Autodesk Inventor part; units mm, degrees
ref_plane "YZ Plane" through (0, 0, 0) normal (1, 0, 0) x (0, 1, 0)
ref_plane "XZ Plane" through (0, 0, 0) normal (0, 1, 0) x (-1, 0, 0)
ref_plane "XY Plane" through (0, 0, 0) normal (0, 0, 1) x (1, 0, 0)
sketch "Skizze1" plane through (0, 0, 0) normal (0, 0, 1) x (1, 0, 0)
  line L0 (0, 0) -> (15, 0)
  line L1 (15, 0) -> (15, -25)
  line L2 (15, -25) -> (0, -25)
  line L3 (0, -25) -> (0, 0)
  line L4 (15.813, -10.2189) -> (15.812, -10.2179)
  line L5 (15.8113, -10.2187) -> (15.812, -10.2194)
  line L6 (15.812, -10.2179) -> (15.8113, -10.2187)
  line L7 (15.812, -10.2179) -> (15.8113, -10.2187)
  line L8 (15.812, -10.2179) -> (15.8113, -10.2187)
  line L9 (15.8113, -10.2187) -> (15.812, -10.2194)
  line L10 (15.8113, -10.2187) -> (15.812, -10.2194)
  line L11 (15.813, -10.2189) -> (15.812, -10.2179)
  line L12 (15.813, -10.2189) -> (15.812, -10.2179)
  line L13 (15.812, -10.2179) -> (15.8113, -10.2187)
  line L14 (15.813, -10.2189) -> (15.812, -10.2179)
  line L15 (15.8113, -10.2187) -> (15.812, -10.2194)
  line L16 (7.5, -8.2332) -> (4.7, -6.6166)
  line L17 (4.7, -6.6166) -> (4.7, -3.3834)
  line L18 (4.7, -3.3834) -> (7.5, -1.7668)
  line L19 (7.5, -1.7668) -> (10.3, -3.3834)
  line L20 (10.3, -3.3834) -> (10.3, -6.6166)
  line L21 (10.3, -6.6166) -> (7.5, -8.2332)
  circle A0 centre (7.5, -5) radius 1.6
  line L22 (10.3, -18.3834) -> (10.3, -21.6166)
  line L23 (10.3, -21.6166) -> (7.5, -23.2332)
  line L24 (7.5, -23.2332) -> (4.7, -21.6166)
  circle A1 centre (7.5, -20) radius 1.6
  line L25 (7.5, -16.7668) -> (10.3, -18.3834)
  line L26 (4.7, -18.3834) -> (7.5, -16.7668)
  line L27 (4.7, -21.6166) -> (4.7, -18.3834)
  dimension "d0" = 25
  dimension "d1" = 15
  dimension "d2" = 5.6
  dimension "d5" = 3.2
  dimension "d6" = 5.6
  dimension "d7" = 3.2
  dimension "d8" = 5
  dimension "d9" = 5
  dimension "d10" = 7.5
extrude "Extrusion1" add sketch "Skizze1" along normal blind 6 contours L0 L1 L2 L3
extrude "Extrusion2" add sketch "Skizze1" along normal blind 3 contours L0 L1 L2 L3 | L16 L17 L18 L19 L20 L21 | L22 L23 L24 L27 L26 L25
equation "\"d9\" = d8"
properties part number "Dribbler Motor Mount Upper Section"
Work out the finished part from the listing and answer in its coordinate system (mm). A direction names the side the tool comes from. Give positions to 0.01 mm unless a question says otherwise; leave off trailing zeros. Loops run counter-clockwise (first coordinate to the right, second up) from the corner with the lowest first, then second, coordinate; pieces in that order, holes last. Notation, with made-up numbers: (-21, -30) - (3, -30) arc R22 cw to (3, -10) - close; hole circle Ø6 at (34, 13.25). An arc over 180 degrees is marked (long way). Answer in a Markdown table with one row per item.
(1) Consider L1, parallel to Y at x = 7.5, z = 1.8; L2, parallel to Y at x = 6.5, z = 3.65; L3, parallel to X at y = -18.75, z = 1.65. Determine where each line is inside the solid, lowest interval first. Write a range as [from, to].
Results list:
| item | result |
|---|---|
| L1 | y = [-25, -21.6], [-18.4, -6.6], [-3.4, 0] |
| L2 | y = [-25, -22.66], [-17.34, -7.66], [-2.34, 0] |
| L3 | x = [0, 6.5], [8.5, 15] |
(2) For a pull along X with two mould halves and no side action, classify faces 3 (the face through (0, -13, 3)), 4 (the face through (6.08, -17.586, 4.479)), 5 (the face through (15, -12, 3)) as pulls with the +X half, pulls with the -X half, needs draft (parallel to the pull), parting line crosses it, or undercut.
Results list:
| item | result |
|---|---|
| face 3 | pulls with the -X half |
| face 4 | undercut |
| face 5 | pulls with the +X half |
(3) Section B-B (z = 3.25) is taken. Give the vertices of the cut face in (x, y), and give its area (3 significant figures).
Results list:
| item | result |
|---|---|
| outline | (0, -25) - (15, -25) - (15, 0) - (0, 0) - close; hole (4.7, -21.62) - (7.5, -23.23) - (10.3, -21.62) - (10.3, -18.38) - (7.5, -16.77) - (4.7, -18.38) - close; hole (4.7, -6.62) - (7.5, -8.23) - (10.3, -6.62) - (10.3, -3.38) - (7.5, -1.77) - (4.7, -3.38) - close |
| area | 321 mm² |
(4) A tool of negligible diameter and unlimited length cuts with its end or side. For faces 1 (the face through (6.08, -2.586, 4.479)), 2 (the face through (6.23, -4.03, 1.48)), from which of +Z, -Z, +X, -X, +Y, -Y can it reach the whole face along a straight path? Write none if from no direction.
Results list:
| item | result |
|---|---|
| face 1 | +Z |
| face 2 | +Z, -Z |
(5) Flat-ended cylindrical pins translate along their axes: pin 1 Ø2.5 at (x, y) = (7.5, -5) entering from +Z; pin 2 Ø1 at (x, z) = (2, 3) entering from +Y; pin 3 Ø3 at (x, y) = (8, -21) entering from +Z. Find the tip coordinate at first contact, or state that the pin passes through.
Results list:
| item | result |
|---|---|
| pin 1 | passes through |
| pin 2 | stops at y = 0 |
| pin 3 | stops at z = 3 |
(6) Section A-A (y = -5) is taken. Give the vertices of the cut face in (x, z), and give its area (3 significant figures).
Results list:
| item | result |
|---|---|
| outline | (0, 0) - (5.9, 0) - (5.9, 3) - (4.7, 3) - (4.7, 6) - (0, 6) - close; (9.1, 0) - (15, 0) - (15, 6) - (10.3, 6) - (10.3, 3) - (9.1, 3) - close |
| area | 63.6 mm² |
(7) Section C-C (y = -22.5) is taken. Give the vertices of the cut face in (x, z).
Results list:
| item | result |
|---|---|
| outline | (0, 0) - (15, 0) - (15, 6) - (8.77, 6) - (8.77, 3) - (6.23, 3) - (6.23, 6) - (0, 6) - close |
(8) Section D-D (y = -19) is taken. Give the vertices of the cut face in (x, z), and give its area (3 significant figures).
Results list:
| item | result |
|---|---|
| outline | (0, 0) - (6.25, 0) - (6.25, 3) - (4.7, 3) - (4.7, 6) - (0, 6) - close; (8.75, 0) - (15, 0) - (15, 6) - (10.3, 6) - (10.3, 3) - (8.75, 3) - close |
| area | 65.7 mm² |
